from build123d import *

# Parameters (mm, degrees)
SKETCH_W               = 82
SKETCH_H               = 100
SKETCH_W_2             = 78
SKETCH_H_2             = 80
PAD_DEPTH              = 2
SKETCH001_W            = 82
SKETCH001_H            = 100
SKETCH001_W_2          = 78
SKETCH001_H_2          = 96
PAD001_DEPTH           = 40
SKETCH002_R            = 6.5
SKETCH002_W            = 5
SKETCH002_H            = 10
POCKET_DEPTH           = 5
SKETCH003_W            = 82
SKETCH003_H            = 100
PAD002_DEPTH           = 2
SKETCH004_W            = 15
SKETCH004_H            = 18
POCKET001_DEPTH        = 5
SKETCH005_R            = 1
PAD003_DEPTH           = 10
POCKET002_DEPTH        = 5
LINEARPATTERN_COUNT    = 5
LINEARPATTERN_PITCH    = 14.75
SKETCH007_W            = 12
SKETCH007_H            = 12
POCKET003_DEPTH        = 5
POCKET004_DEPTH        = 5
LINEARPATTERN001_COUNT = 6
LINEARPATTERN001_PITCH = 12
SKETCH009_R            = 1
PAD004_DEPTH           = 10
SKETCH010_R            = 1.3
SKETCH010_W            = 70
SKETCH010_H            = 8
POCKET005_DEPTH        = 3


with BuildPart() as part:
    # Sketch → Pad (new body)
    with BuildSketch(Plane.XY):
        with Locations((41, -50)):
            Rectangle(SKETCH_W, SKETCH_H)
        with Locations((41, -50)):
            Rectangle(SKETCH_W_2, SKETCH_H_2, mode=Mode.SUBTRACT)
    extrude(amount=PAD_DEPTH)

    # Sketch001 (on Face10 of Pad) → Pad001 (join)
    with BuildSketch(Plane.XY.offset(2)):
        with Locations((41, -50)):
            Rectangle(SKETCH001_W, SKETCH001_H)
        with Locations((41, -50)):
            Rectangle(SKETCH001_W_2, SKETCH001_H_2, mode=Mode.SUBTRACT)
    extrude(amount=PAD001_DEPTH)

    # Sketch002 (on Face8 of Pad001) → Pocket (cut)
    with BuildSketch(Plane.YZ.offset(82)):
        with Locations((-60, 22)):
            Circle(SKETCH002_R)
        with Locations((-35, 22)):
            Circle(SKETCH002_R)
        with Locations((-4.5, 22)):
            Rectangle(SKETCH002_W, SKETCH002_H)
    extrude(amount=-POCKET_DEPTH, mode=Mode.SUBTRACT)

    # Sketch003 (on Face13 of Pocket) → Pad002 (join)
    with BuildSketch(Plane.XY.offset(42)):
        with Locations((41, -50)):
            Rectangle(SKETCH003_W, SKETCH003_H)
    extrude(amount=PAD002_DEPTH)

    # Sketch004 (on Face5 of Pad002) → Pocket001 (cut)
    with BuildSketch(Plane.XZ.offset(100)):
        with BuildLine():
            ThreePointArc((45, 18), (42, 15), (45, 12))
            Line((45, 12), (70, 12))
            ThreePointArc((70, 12), (73, 15), (70, 18))
            Line((45, 18), (70, 18))
        make_face()
        with Locations((10.5, 22)):
            Rectangle(SKETCH004_W, SKETCH004_H)
    extrude(amount=-POCKET001_DEPTH, mode=Mode.SUBTRACT)

    # Sketch005 (on Face7 of Pocket001) → Pad003 (join)
    with BuildSketch(Plane(origin=(0, 0, 0), x_dir=(0, -1, 0), z_dir=(-1, 0, 0))):
        with Locations((96, 34)):
            Circle(SKETCH005_R)
        with Locations((96, 11)):
            Circle(SKETCH005_R)
    extrude(amount=-PAD003_DEPTH)

    # Sketch006 (on Face22 of Pad003) → Pocket002 (cut)
    with BuildSketch(Plane(origin=(0, 0, 0), x_dir=(-1, 0, 0), z_dir=(0, 1, 0))):
        with BuildLine():
            ThreePointArc((-75, 11), (-76, 10), (-75, 9))
            Line((-75, 9), (-70, 9))
            ThreePointArc((-70, 9), (-69, 10), (-70, 11))
            Line((-75, 11), (-70, 11))
        make_face()
        with BuildLine():
            ThreePointArc((-75, 36), (-76, 35), (-75, 34))
            Line((-75, 34), (-70, 34))
            ThreePointArc((-70, 34), (-69, 35), (-70, 36))
            Line((-75, 36), (-70, 36))
        make_face()
    pocket002 = extrude(amount=-POCKET002_DEPTH, mode=Mode.SUBTRACT)

    # LinearPattern: Pocket002 ×5
    with Locations(*[(-i * LINEARPATTERN_PITCH, 0, 0) for i in range(1, LINEARPATTERN_COUNT)]):
        add(pocket002, mode=Mode.SUBTRACT)

    # Sketch007 (on Face22 of LinearPattern) → Pocket003 (cut)
    with BuildSketch(Plane(origin=(0, 0, 0), x_dir=(-1, 0, 0), z_dir=(0, 1, 0))):
        with Locations((-14, 25)):
            Rectangle(SKETCH007_W, SKETCH007_H)
    extrude(amount=-POCKET003_DEPTH, mode=Mode.SUBTRACT)

    # Sketch008 (on Face37 of Pocket003) → Pocket004 (cut)
    with BuildSketch(Plane.XY.offset(44)):
        with BuildLine():
            ThreePointArc((12, -10), (10, -8), (8, -10))
            Line((8, -10), (8, -90))
            ThreePointArc((8, -90), (10, -92), (12, -90))
            Line((12, -10), (12, -90))
        make_face()
    pocket004 = extrude(amount=-POCKET004_DEPTH, mode=Mode.SUBTRACT)

    # LinearPattern001: Pocket004 ×6
    with Locations(*[(i * LINEARPATTERN001_PITCH, 0, 0) for i in range(1, LINEARPATTERN001_COUNT)]):
        add(pocket004, mode=Mode.SUBTRACT)

    # Sketch009 (on Face37 of LinearPattern001) → Pad004 (join)
    with BuildSketch(Plane.XY.offset(44)):
        with Locations((54, -40)):
            Circle(SKETCH009_R)
        with Locations((38, -40)):
            Circle(SKETCH009_R)
        with Locations((38, -85)):
            Circle(SKETCH009_R)
        with Locations((54, -85)):
            Circle(SKETCH009_R)
    extrude(amount=-PAD004_DEPTH)

    # Sketch010 (on Face4 of Pad004) → Pocket005 (cut)
    with BuildSketch(Plane(origin=(0, 0, 0), x_dir=(1, 0, 0), z_dir=(0, 0, -1))):
        with Locations((4, 4)):
            Circle(SKETCH010_R)
        with Locations((78, 96)):
            Circle(SKETCH010_R)
        with Locations((45, 6)):
            Rectangle(SKETCH010_W, SKETCH010_H)
        with Locations((37, 94)):
            Rectangle(SKETCH010_W, SKETCH010_H)
    extrude(amount=-POCKET005_DEPTH, mode=Mode.SUBTRACT)


solid = part.part
Geometry: final body of the model. Coordinates: model frame, mm. A direction names the side the tool comes from. Round coordinates to 2 decimals unless told otherwise and drop trailing zeros. Order: outer loops, then holes, each group sorted by start corner. A loop starts at its lowest first (then second) coordinate and runs counter-clockwise, first axis right, second up.
Q1. Section D-D, the plane x = 78. Output: boundary loops of the cut face in (y, z).
Result sheet:
outline: (-100, 0) - (-97.3, 0) - (-97.3, 2) - (-98, 2) - (-98, 42) - (-2, 42) - (-2, 0) - (0, 0) - (0, 44) - (-100, 44) - close; (-94.7, 0) - (-90, 0) - (-90, 2) - (-94.7, 2) - close
Q2. Section C-C, the plane y = -52. Give the number of separate pieces and of enclosed holes in the cut face, and give its area (3 significant figures).
Result sheet:
separate pieces: 7
enclosed holes: 0
area: 284 mm2
Q3. Mould query, pull axis Y, two halves, no side actions, for faces 6 (the face through (40.8, -1.6, 0)), 7 (the face through (80, -51, 21)), 8 (the face through (40, 0, 22)), 9 (the face through (40, -100, 22)). Classes: released by +Y, released by -Y, zero draft, split by the parting line, or undercut.
Result sheet:
face 6: zero draft
face 7: undercut
face 8: released by +Y
face 9: released by -Y
Q4. Section B-B, the plane x = 34. Output: boundary loops of the cut face in (y, z).
Result sheet:
outline: (-100, 0) - (-98, 0) - (-98, 42) - (-92, 42) - (-92, 44) - (-100, 44) - close; (-8, 42) - (-2, 42) - (-2, 0) - (0, 0) - (0, 44) - (-8, 44) - close
Q5. Pin query (flat end, axial travel): pin 1 (2 mm diameter, centred on x = 18, y = -65, fed in from -Z); pin 2 (1.5 mm diameter, centred on x = 9, z = 14, fed in from -Y). Return the tip coordinate at first contact, or that it passes through.
Result sheet:
pin 1: stops at z = 42
pin 2: stops at y = -2
Q6. Material intervals for probe 1 along X at (y, z) = (-21, 39.5); probe 2 along Y at (x, z) = (15, 5); probe 3 along Z at (x, y) = (72.5, -95), sorted ascending.
Result sheet:
probe 1: x = 0 to 2, 80 to 82
probe 2: y = -100 to -98, -2 to 0
probe 3: z = 0 to 2, 42 to 44
Q7. Section A-A, the plane z = 6.5. Output: boundary loops of the cut face in (x, y).
Result sheet:
outline: (0, -100) - (82, -100) - (82, 0) - (0, 0) - close; hole (2, -98) - (80, -98) - (80, -2) - (2, -2) - close
Q8. Access query for faces 1 (the face through (79.2, -95.5, 1)), 2 (the face through (81.01, -53.8, 23.95)), 3 (the face through (0, -49, 22)), 4 (the face through (6, -6, 2)), 5 (the face through (42, -99, 15)). Directions: +Z, -Z, +X, -X, +Y, -Y. A direction counts if a zero-diameter tool reaches every point of the face in a straight line with its end or side. Return the directions, or none.
Result sheet:
face 1: -Z
face 2: +X
face 3: +Z, -Z, -X, +Y, -Y
face 4: none
face 5: -Y
